Verification items for the finished model (mm, model axes). A direction names the side the tool comes from. Round coordinates to 2 decimals unless told otherwise and drop trailing zeros. Order: outer loops, then holes, each group sorted by start corner. A loop starts at its lowest first (then second) coordinate and runs counter-clockwise, first axis right, second up. Notation, with made-up numbers: (-23.75, -29.75) -> (14.25, -29.75) arc R3 cw to (14.25, -24.75) -> close; hole circle Ø11 at (-6.5, 82). An arc over 180 degrees is marked (long way). Return JSON: item names as keys, results as strings. Group by question number.
1) Section check C-C on z = 10. Enter the section's corners in (x, y).
2) Depth check by flat-ended pin: pin 1 (3 mm diameter, centred on x = 8, y = 0, fed in from +Z); pin 2 (2 mm diameter, centred on x = 0, y = -6, fed in from +Z); pin 3 (1 mm diameter, centred on x = -1, y = -9, fed in from -Z). Enter the tip coordinate at first touch or a pass-through.
3) Section check A-A on y = 0. Enter the section's corners in (x, z).
4) Scan lines: L1, parallel to Y at x = 0, z = 1.5 (3 decimals); L2, parallel to Y at x = 0, z = 0.85; L3, parallel to Z at x = 1, y = 8.5. Record each from-to range of solid material in increasing order.
5) Section check B-B on x = 0. Enter the section's corners in (y, z).
6) Section check D-D on z = 22.5. Enter the section's corners in (x, y), plus the area to 3 significant figures.
7) Tool access check on faces 4 (the cylindrical face through (-7.25, 0.05, 25.61)), 5 (the flat face through (0, 10, 3)), 6 (the flat face through (0, 0, 0)). Record the directions out of +Z, -Z, +X, -X, +Y, -Y that give a thin tool (end or side, any length) a straight path to the whole face; none if there is none.
8) Draft check along X on faces 1 (the cylindrical face through (-3.02, -13.62, 12.92)), 2 (the flat face through (0, 6, 24.09)), 3 (the flat face through (0, 0, 29.34)). Enter one of: pulls with the +X half, pulls with the -X half, needs draft (parallel to the pull), parting line crosses it, or undercut.
```python
from build123d import *

# Parameters (mm, degrees)
SKETCH1_R           = 13.95
BOSS_EXTRUDE1_DEPTH = 29.34
SKETCH2_R           = 13.95
SKETCH2_R_2         = 4.42
CUT_EXTRUDE1_DEPTH  = 2.25
CHAMFER1_SIZE       = 5
CHAMFER1_SIZE2      = 4.5
CHAMFER2_SIZE       = 1
CHAMFER2_SIZE2      = 4
SKETCH3_R           = 1.75
CUT_EXTRUDE2_DEPTH  = 3
SKETCH4_R           = 1.25
CUT_EXTRUDE3_DEPTH  = 3


with BuildPart() as part:
    # Sketch1 → Boss-Extrude1 (new body)
    with BuildSketch(Plane.XY):
        Circle(SKETCH1_R)
    extrude(amount=BOSS_EXTRUDE1_DEPTH)

    # Sketch2 → Cut-Extrude1 (cut)
    with BuildSketch(Plane.XY.offset(29.34)):
        Circle(SKETCH2_R)
        Circle(SKETCH2_R_2, mode=Mode.SUBTRACT)
    extrude(amount=-CUT_EXTRUDE1_DEPTH, mode=Mode.SUBTRACT)

    # Chamfer1
    chamfer1_edges = [part.edges().sort_by_distance(p)[0] for p in [
        (-13.95, 0, 27.09),
    ]]
    chamfer1_side = [part.faces().sort_by_distance(p)[0] for p in [
        (-13.95, 0, 13.545),
    ]]
    chamfer(chamfer1_edges, length=CHAMFER1_SIZE, length2=CHAMFER1_SIZE2, reference=chamfer1_side[0])

    # Chamfer2
    chamfer2_edges = [part.edges().sort_by_distance(p)[0] for p in [
        (-13.95, 0, 0),
    ]]
    chamfer2_side = [part.faces().sort_by_distance(p)[0] for p in [
        (0, 0, 0),
    ]]
    chamfer(chamfer2_edges, length=CHAMFER2_SIZE, length2=CHAMFER2_SIZE2, reference=chamfer2_side[0])

    # Sketch3 → Cut-Extrude2 (cut)
    with BuildSketch(Plane(origin=(0, 0, 0), x_dir=(-1, 0, 0), z_dir=(0, 0, -1))):
        with Locations((8, 0)):
            Circle(SKETCH3_R)
        with Locations((-8, 0)):
            Circle(SKETCH3_R)
        with Locations((0, -9.5)):
            Circle(SKETCH3_R)
        with Locations((0, 9.5)):
            Circle(SKETCH3_R)
    extrude(amount=-CUT_EXTRUDE2_DEPTH, mode=Mode.SUBTRACT)

    # Sketch4 → Cut-Extrude3 (cut)
    with BuildSketch(Plane.XY.offset(27.09)):
        with Locations((0, 6)):
            Circle(SKETCH4_R)
        with Locations((6, 0)):
            Circle(SKETCH4_R)
        with Locations((0, -6)):
            Circle(SKETCH4_R)
        with Locations((-6, 0)):
            Circle(SKETCH4_R)
    extrude(amount=-CUT_EXTRUDE3_DEPTH, mode=Mode.SUBTRACT)


solid = part.part
```
Check result:
{
 "1": {"outline": "circle Ø27.9 at (0, 0)"},
 "2": {"pin 1": "z = 27.09", "pin 2": "z = 24.09", "pin 3": "z = 3"},
 "3": {"outline": "(-13.95, 4) -> (-12.95, 0) -> (-9.75, 0) -> (-9.75, 3) -> (-6.25, 3) -> (-6.25, 0) -> (6.25, 0) -> (6.25, 3) -> (9.75, 3) -> (9.75, 0) -> (12.95, 0) -> (13.95, 4) -> (13.95, 22.09) -> (9.45, 27.09) -> (7.25, 27.09) -> (7.25, 24.09) -> (4.75, 24.09) -> (4.75, 27.09) -> (4.42, 27.09) -> (4.42, 29.34) -> (-4.42, 29.34) -> (-4.42, 27.09) -> (-4.75, 27.09) -> (-4.75, 24.09) -> (-7.25, 24.09) -> (-7.25, 27.09) -> (-9.45, 27.09) -> (-13.95, 22.09) -> close"},
 "4": {"L1": "-13.325 to -11.25, -7.75 to 7.75, 11.25 to 13.325", "L2": "-13.16 to -11.25, -7.75 to 7.75, 11.25 to 13.16", "L3": "3 to 27.09"},
 "5": {"outline": "(-13.95, 4) -> (-12.95, 0) -> (-11.25, 0) -> (-11.25, 3) -> (-7.75, 3) -> (-7.75, 0) -> (7.75, 0) -> (7.75, 3) -> (11.25, 3) -> (11.25, 0) -> (12.95, 0) -> (13.95, 4) -> (13.95, 22.09) -> (9.45, 27.09) -> (7.25, 27.09) -> (7.25, 24.09) -> (4.75, 24.09) -> (4.75, 27.09) -> (4.42, 27.09) -> (4.42, 29.34) -> (-4.42, 29.34) -> (-4.42, 27.09) -> (-4.75, 27.09) -> (-4.75, 24.09) -> (-7.25, 24.09) -> (-7.25, 27.09) -> (-9.45, 27.09) -> (-13.95, 22.09) -> close"},
 "6": {"outline": "circle Ø27.16 at (0, 0)", "area": "579 mm^2"},
 "7": {"face 4": "+Z", "face 5": "-Z", "face 6": "-Z, +X, -X, +Y, -Y"},
 "8": {"face 1": "parting line crosses it", "face 2": "undercut", "face 3": "needs draft"}
}
